Read the model definition and answer for the solid it produces. Units are mm, in the model's axes. A direction names the side the tool comes from. Coordinates: 2 decimals unless noted, no trailing zeros. Loops run counter-clockwise (first coordinate to the right, second up) from the corner with the lowest first, then second, coordinate; pieces in that order, holes last.
Q1. Section D-D (y = -5) is taken. Give the vertices of the cut face in (x, z).
Q2. Section C-C (x = 6.5) is taken. Give the vertices of the cut face in (y, z).
Q3. Straight lines are drawn through the part: line 1 (Z direction, x = -2, y = 0); line 2 (X direction, y = -20.5, z = 4); line 3 (Z direction, x = -4, y = 18). For each, find the intervals that lie inside material, in ascending order.
Q4. Section A-A (y = 0) is taken. Give the vertices of the cut face in (x, z), then the cut area to 3 significant figures.
Q5. Flat-ended cylindrical pins translate along their axes: P1, Ø6, axis at y = -13, z = 32.5, coming from the +X side; P2, Ø4.5, axis at x = 0, y = -0.5, coming from the +Z side. Find the tip coordinate at first contact, or state that the pin passes through.
Q6. Section B-B (z = 21) is taken. Give the vertices of the cut face in (x, y).
Q7. The mould has two halves that part along X. Classify faces 4 (the face through (-8.1, 17.51, 12.97)), 5 (the face through (10, 0, 15)), 6 (the face through (7.5, 0, 12)): pulls with the +X half, pulls with the -X half, needs draft (parallel to the pull), parting line crosses it, or undercut.
Q8. Which of the six approach directions +Z, -Z, +X, -X, +Y, -Y give full straight-line access (tool end or side, diameter ignored) to faces 1 (the face through (0, 0, 2.5)), 2 (the face through (-0.105, -1.244, 24.705)), 3 (the face through (-10, 0, 15))?
from build123d import *

# Parameters (mm, degrees)
F0_R     = 3.238814
F1_DEPTH = 10
F2_T     = -2.5


with BuildPart() as f1:
    # F0 (on Right) → F1 (new body, symmetric)
    with BuildSketch(Plane.YZ):
        with BuildLine():
            Line((-25, 0), (0, 0))
            Line((0, 0), (25, 0))
            Line((25, 0), (5.626596, 33.55572))
            ThreePointArc((5.626596, 33.55572), (0, 36.804237), (-5.626596, 33.55572))
            Line((-5.626596, 33.55572), (-25, 0))
        make_face()
        with Locations((0, 30.307204)):
            Circle(F0_R, mode=Mode.SUBTRACT)
    extrude(amount=F1_DEPTH, both=True)

    # F2
    f2_openings = [f1.faces().sort_by_distance(p)[0] for p in [
        (0, 15.313298, 16.77786),
        (0, -15.313298, 16.77786),
        (0, 0, 36.804237),
    ]]
    offset(amount=F2_T, openings=f2_openings)


solid = f1.part
Numbers:
1. outline: (-10, 0) - (10, 0) - (10, 34.46) - (7.5, 34.46) - (7.5, 33.12) - (-7.5, 33.12) - (-7.5, 34.46) - (-10, 34.46) - close; hole (-7.5, 2.5) - (7.5, 2.5) - (7.5, 27.49) - (-7.5, 27.49) - close
2. outline: (-25, 0) - (25, 0) - (23.56, 2.5) - (-23.56, 2.5) - close; circle Ø11.48 at (0, 30.31); hole circle Ø6.48 at (0, 30.31)
3. line 1: z = 0 to 2.5, 24.57 to 27.07, 33.55 to 36.05
3. line 2: x = -10 to -7.5, 7.5 to 10
3. line 3: z = 0 to 2.5
4. outline: (-10, 0) - (10, 0) - (10, 27.07) - (-10, 27.07) - close; (-10, 33.55) - (10, 33.55) - (10, 36.8) - (7.5, 36.8) - (7.5, 36.05) - (-7.5, 36.05) - (-7.5, 36.8) - (-10, 36.8) - close; hole (-7.5, 2.5) - (7.5, 2.5) - (7.5, 24.57) - (-7.5, 24.57) - close
4. area: 264 mm2
5. P1: passes through
5. P2: stops at z = 36.05
6. outline: (-10, -12.88) - (-7.5, -12.88) - (-7.5, 12.88) - (-10, 12.88) - close; (7.5, -12.88) - (10, -12.88) - (10, 12.88) - (7.5, 12.88) - close
7. face 4: needs draft
7. face 5: pulls with the +X half
7. face 6: undercut
8. face 1: +Y, -Y
8. face 2: none
8. face 3: +Z, -Z, -X, +Y, -Y
